Geometry check sheet. Reference: the model listing, model coordinates, mm. Round coordinates to 2 decimals unless told otherwise and drop trailing zeros. Write each loop counter-clockwise with the first axis right and the second up, starting at its lowest first coordinate (ties: lowest second). Pieces come first, ordered by that corner, then holes.
Item 1: Depth check by flat-ended pin: P1, Ø1, axis at y = 24.5, z = -292.5, coming from the -X side; P2, Ø1, axis at y = 2, z = -225, coming from the -X side; P3, Ø3.5, axis at y = 21.5, z = -232, coming from the +X side. Enter the tip coordinate at first touch or a pass-through.
Item 2: Cross-section at C-C (z = -63.5). State how many separate pieces and enclosed holes the cut face has, then the cut area to 3 significant figures.
Item 3: Scan lines: probe 1 along X at (y, z) = (34, -332); probe 2 along Y at (x, z) = (20, -145); probe 3 along X at (y, z) = (14.5, -21). Record each from-to range of solid material in increasing order.
Item 4: Cross-section at A-A (x = 20). Enter the section's corners in (y, z), then the cut area to 4 significant figures.
from build123d import *

# Parameters (mm, degrees)
SKETCH1_R           = 3.4
BOSS_EXTRUDE1_DEPTH = 350


with BuildPart() as part:
    # Sketch1 → Boss-Extrude1 (new body)
    with BuildSketch(Plane.XY):
        with BuildLine():
            Line((0, 36), (0, 25.5))
            ThreePointArc((0, 25.5), (0.439339828, 24.439339828), (1.5, 24))
            Line((1.5, 24), (3.5, 24))
            ThreePointArc((3.5, 24), (4.207106781, 24.292893219), (4.5, 25))
            Line((4.5, 25), (4.5, 26.5))
            ThreePointArc((4.5, 26.5), (4.353553391, 26.853553391), (4, 27))
            Line((4, 27), (2.5, 27))
            ThreePointArc((2.5, 27), (2.146446609, 27.146446609), (2, 27.5))
            ThreePointArc((2, 27.5), (2.732233047, 29.267766953), (4.5, 30))
            Line((4.5, 30), (5.807611845, 30))
            ThreePointArc((5.807611845, 30), (7.721029006, 29.619397663), (9.343145751, 28.535533906))
            Line((9.343145751, 28.535533906), (10.785533906, 27.093145751))
            ThreePointArc((10.785533906, 27.093145751), (11.869397663, 25.471029006), (12.25, 23.557611845))
            Line((12.25, 23.557611845), (12.25, 16.442388155))
            ThreePointArc((12.25, 16.442388155), (11.869397663, 14.528970994), (10.785533906, 12.906854249))
            Line((10.785533906, 12.906854249), (9.343145751, 11.464466094))
            ThreePointArc((9.343145751, 11.464466094), (7.721029006, 10.380602337), (5.807611845, 10))
            Line((5.807611845, 10), (4.5, 10))
            ThreePointArc((4.5, 10), (2.732233047, 10.732233047), (2, 12.5))
            ThreePointArc((2, 12.5), (2.146446609, 12.853553391), (2.5, 13))
            Line((2.5, 13), (4, 13))
            ThreePointArc((4, 13), (4.353553391, 13.146446609), (4.5, 13.5))
            Line((4.5, 13.5), (4.5, 15))
            ThreePointArc((4.5, 15), (4.207106781, 15.707106781), (3.5, 16))
            Line((3.5, 16), (1.5, 16))
            ThreePointArc((1.5, 16), (0.439339828, 15.560660172), (0, 14.5))
            Line((0, 14.5), (0, 4))
            ThreePointArc((0, 4), (1.171572875, 1.171572875), (4, 0))
            Line((4, 0), (14.5, 0))
            ThreePointArc((14.5, 0), (15.560660172, 0.439339828), (16, 1.5))
            Line((16, 1.5), (16, 3.5))
            ThreePointArc((16, 3.5), (15.707106781, 4.207106781), (15, 4.5))
            Line((15, 4.5), (13.5, 4.5))
            ThreePointArc((13.5, 4.5), (13.146446609, 4.353553391), (13, 4))
            Line((13, 4), (13, 2.5))
            ThreePointArc((13, 2.5), (12.853553391, 2.146446609), (12.5, 2))
            ThreePointArc((12.5, 2), (10.732233047, 2.732233047), (10, 4.5))
            Line((10, 4.5), (10, 5.807611845))
            ThreePointArc((10, 5.807611845), (10.380602337, 7.721029006), (11.464466094, 9.343145751))
            Line((11.464466094, 9.343145751), (12.906854249, 10.785533906))
            ThreePointArc((12.906854249, 10.785533906), (14.528970994, 11.869397663), (16.442388155, 12.25))
            Line((16.442388155, 12.25), (23.557611845, 12.25))
            ThreePointArc((23.557611845, 12.25), (25.471029006, 11.869397663), (27.093145751, 10.785533906))
            Line((27.093145751, 10.785533906), (28.535533906, 9.343145751))
            ThreePointArc((28.535533906, 9.343145751), (29.619397663, 7.721029006), (30, 5.807611845))
            Line((30, 5.807611845), (30, 4.5))
            ThreePointArc((30, 4.5), (29.267766953, 2.732233047), (27.5, 2))
            ThreePointArc((27.5, 2), (27.146446609, 2.146446609), (27, 2.5))
            Line((27, 2.5), (27, 4))
            ThreePointArc((27, 4), (26.853553391, 4.353553391), (26.5, 4.5))
            Line((26.5, 4.5), (25, 4.5))
            ThreePointArc((25, 4.5), (24.292893219, 4.207106781), (24, 3.5))
            Line((24, 3.5), (24, 1.5))
            ThreePointArc((24, 1.5), (24.439339828, 0.439339828), (25.5, 0))
            Line((25.5, 0), (36, 0))
            ThreePointArc((36, 0), (38.828427125, 1.171572875), (40, 4))
            Line((40, 4), (40, 14.5))
            ThreePointArc((40, 14.5), (39.560660172, 15.560660172), (38.5, 16))
            Line((38.5, 16), (36.5, 16))
            ThreePointArc((36.5, 16), (35.792893219, 15.707106781), (35.5, 15))
            Line((35.5, 15), (35.5, 13.5))
            ThreePointArc((35.5, 13.5), (35.646446609, 13.146446609), (36, 13))
            Line((36, 13), (37.5, 13))
            ThreePointArc((37.5, 13), (37.853553391, 12.853553391), (38, 12.5))
            ThreePointArc((38, 12.5), (37.267766953, 10.732233047), (35.5, 10))
            Line((35.5, 10), (34.192388155, 10))
            ThreePointArc((34.192388155, 10), (32.278970994, 10.380602337), (30.656854249, 11.464466094))
            Line((30.656854249, 11.464466094), (29.214466094, 12.906854249))
            ThreePointArc((29.214466094, 12.906854249), (28.130602337, 14.528970994), (27.75, 16.442388155))
            Line((27.75, 16.442388155), (27.75, 23.557611845))
            ThreePointArc((27.75, 23.557611845), (28.130602337, 25.471029006), (29.214466094, 27.093145751))
            Line((29.214466094, 27.093145751), (30.656854249, 28.535533906))
            ThreePointArc((30.656854249, 28.535533906), (32.278970994, 29.619397663), (34.192388155, 30))
            Line((34.192388155, 30), (35.5, 30))
            ThreePointArc((35.5, 30), (37.267766953, 29.267766953), (38, 27.5))
            ThreePointArc((38, 27.5), (37.853553391, 27.146446609), (37.5, 27))
            Line((37.5, 27), (36, 27))
            ThreePointArc((36, 27), (35.646446609, 26.853553391), (35.5, 26.5))
            Line((35.5, 26.5), (35.5, 25))
            ThreePointArc((35.5, 25), (35.792893219, 24.292893219), (36.5, 24))
            Line((36.5, 24), (38.5, 24))
            ThreePointArc((38.5, 24), (39.560660172, 24.439339828), (40, 25.5))
            Line((40, 25.5), (40, 36))
            ThreePointArc((40, 36), (38.828427125, 38.828427125), (36, 40))
            Line((36, 40), (25.5, 40))
            ThreePointArc((25.5, 40), (24.439339828, 39.560660172), (24, 38.5))
            Line((24, 38.5), (24, 36.5))
            ThreePointArc((24, 36.5), (24.292893219, 35.792893219), (25, 35.5))
            Line((25, 35.5), (26.5, 35.5))
            ThreePointArc((26.5, 35.5), (26.853553391, 35.646446609), (27, 36))
            Line((27, 36), (27, 37.5))
            ThreePointArc((27, 37.5), (27.146446609, 37.853553391), (27.5, 38))
            ThreePointArc((27.5, 38), (29.267766953, 37.267766953), (30, 35.5))
            Line((30, 35.5), (30, 34.192388155))
            ThreePointArc((30, 34.192388155), (29.619397663, 32.278970994), (28.535533906, 30.656854249))
            Line((28.535533906, 30.656854249), (27.093145751, 29.214466094))
            ThreePointArc((27.093145751, 29.214466094), (25.471029006, 28.130602337), (23.557611845, 27.75))
            Line((23.557611845, 27.75), (16.442388155, 27.75))
            ThreePointArc((16.442388155, 27.75), (14.528970994, 28.130602337), (12.906854249, 29.214466094))
            Line((12.906854249, 29.214466094), (11.464466094, 30.656854249))
            ThreePointArc((11.464466094, 30.656854249), (10.380602337, 32.278970994), (10, 34.192388155))
            Line((10, 34.192388155), (10, 35.5))
            ThreePointArc((10, 35.5), (10.732233047, 37.267766953), (12.5, 38))
            ThreePointArc((12.5, 38), (12.853553391, 37.853553391), (13, 37.5))
            Line((13, 37.5), (13, 36))
            ThreePointArc((13, 36), (13.146446609, 35.646446609), (13.5, 35.5))
            Line((13.5, 35.5), (15, 35.5))
            ThreePointArc((15, 35.5), (15.707106781, 35.792893219), (16, 36.5))
            Line((16, 36.5), (16, 38.5))
            ThreePointArc((16, 38.5), (15.560660172, 39.560660172), (14.5, 40))
            Line((14.5, 40), (4, 40))
            ThreePointArc((4, 40), (1.171572875, 38.828427125), (0, 36))
        make_face()
        with Locations(Location((20, 20, 0), (0, 0, 180))):
            Circle(SKETCH1_R, mode=Mode.SUBTRACT)
        with BuildLine():
            Line((1.8, 4), (1.8, 7.7))
            ThreePointArc((1.8, 7.7), (1.946446609, 8.053553391), (2.3, 8.2))
            Line((2.3, 8.2), (7.7, 8.2))
            ThreePointArc((7.7, 8.2), (8.053553391, 8.053553391), (8.2, 7.7))
            Line((8.2, 7.7), (8.2, 2.3))
            ThreePointArc((8.2, 2.3), (8.053553391, 1.946446609), (7.7, 1.8))
            Line((7.7, 1.8), (4, 1.8))
            ThreePointArc((4, 1.8), (2.444365081, 2.444365081), (1.8, 4))
        make_face(mode=Mode.SUBTRACT)
        with BuildLine():
            Line((4, 38.2), (7.7, 38.2))
            ThreePointArc((7.7, 38.2), (8.053553391, 38.053553391), (8.2, 37.7))
            Line((8.2, 37.7), (8.2, 32.3))
            ThreePointArc((8.2, 32.3), (8.053553391, 31.946446609), (7.7, 31.8))
            Line((7.7, 31.8), (2.3, 31.8))
            ThreePointArc((2.3, 31.8), (1.946446609, 31.946446609), (1.8, 32.3))
            Line((1.8, 32.3), (1.8, 36))
            ThreePointArc((1.8, 36), (2.444365081, 37.555634919), (4, 38.2))
        make_face(mode=Mode.SUBTRACT)
        with BuildLine():
            Line((31.8, 32.3), (31.8, 37.7))
            ThreePointArc((31.8, 37.7), (31.946446609, 38.053553391), (32.3, 38.2))
            Line((32.3, 38.2), (36, 38.2))
            ThreePointArc((36, 38.2), (37.555634919, 37.555634919), (38.2, 36))
            Line((38.2, 36), (38.2, 32.3))
            ThreePointArc((38.2, 32.3), (38.053553391, 31.946446609), (37.7, 31.8))
            Line((37.7, 31.8), (32.3, 31.8))
            ThreePointArc((32.3, 31.8), (31.946446609, 31.946446609), (31.8, 32.3))
        make_face(mode=Mode.SUBTRACT)
        with BuildLine():
            Line((32.3, 8.2), (37.7, 8.2))
            ThreePointArc((37.7, 8.2), (38.053553391, 8.053553391), (38.2, 7.7))
            Line((38.2, 7.7), (38.2, 4))
            ThreePointArc((38.2, 4), (37.555634919, 2.444365081), (36, 1.8))
            Line((36, 1.8), (32.3, 1.8))
            ThreePointArc((32.3, 1.8), (31.946446609, 1.946446609), (31.8, 2.3))
            Line((31.8, 2.3), (31.8, 7.7))
            ThreePointArc((31.8, 7.7), (31.946446609, 8.053553391), (32.3, 8.2))
        make_face(mode=Mode.SUBTRACT)
    extrude(amount=-BOSS_EXTRUDE1_DEPTH)


solid = part.part
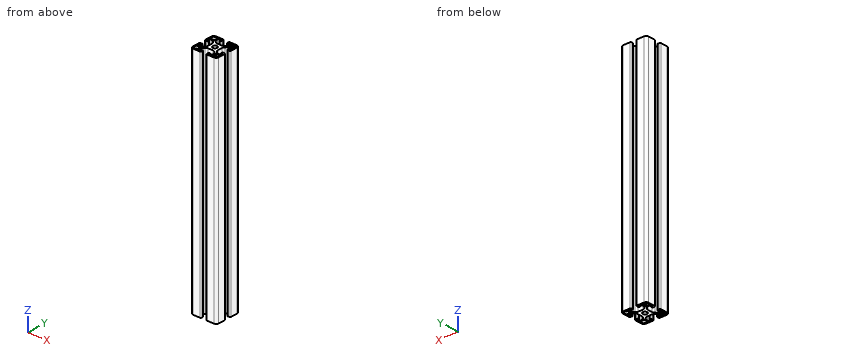
Resolved:
1. P1: stops at x = 0.09
1. P2: stops at x = 0.29
1. P3: stops at x = 27.75
2. separate pieces: 1
2. enclosed holes: 5
2. area: 657 mm2
3. probe 1: x = 0 to 1.8, 8.2 to 10, 30 to 31.8, 38.2 to 40
3. probe 2: y = 12.25 to 16.6, 23.4 to 27.75
3. probe 3: x = 0 to 4.5, 11.86 to 28.14, 35.5 to 40
4. outline: (12.25, -350) - (16.6, -350) - (16.6, 0) - (12.25, 0) - close; (23.4, -350) - (27.75, -350) - (27.75, 0) - (23.4, 0) - close
4. area: 3,045 mm2
